Input: dimensioned drawing with shaded views. Units: mm. Origin: part minimum x, y, z. A direction names the side the tool comes from. Round coordinates to 2 decimals unless told otherwise and drop trailing zeros. Loops run counter-clockwise (first coordinate to the right, second up) from the corner with the lowest first, then second, coordinate; pieces in that order, holes last. Notation, with made-up numbers: M 88.5,0.25 L 146.5,0.25 A5 cw 146.5,8.25 Z; hole C 55.25,47 d4. An arc over 180 degrees is marked long. Answer as CSV lines item,"result". Start each with the question number.
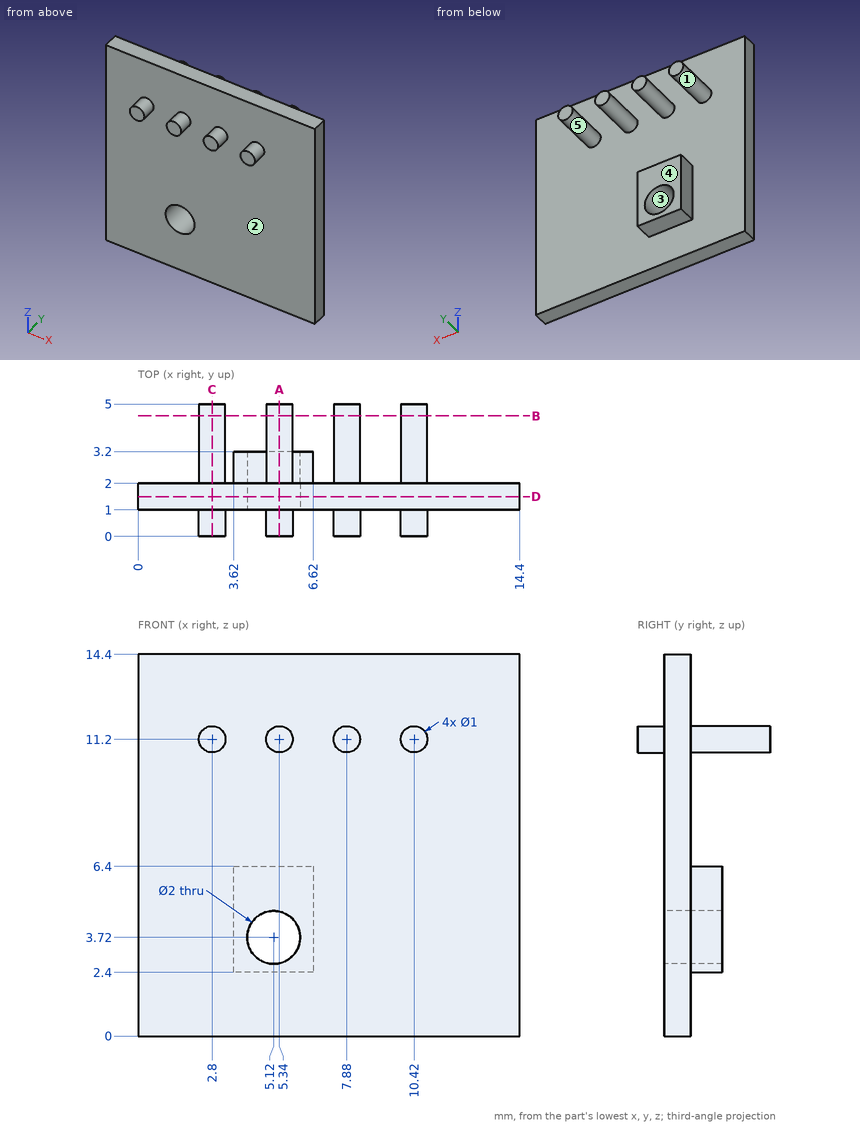
1) Contact query for flat-ended pins moving along their axis: pin 1 Ø1.3 at (y, z) = (3, 4.5) entering from +X; pin 2 Ø3 at (x, y) = (11, 4) entering from +Z; pin 3 Ø1.5 at (x, z) = (11, 3.5) entering from +Y. Output: stop coordinate, or through.
2) Ray query, line 1 along Z through (x, y) = (5.12, 2.1); line 2 along Y through (x, z) = (7, 11); line 3 along Y through (x, z) = (6.5, 5.5). Return the intervals inside material, ascending.
3) Mould query, pull axis Z, two halves, no side actions, for the marked faces 1, 2 and 3. Classes: pulls with the +Z half, pulls with the -Z half, needs draft (parallel to the pull), parting line crosses it, or undercut.
4) Section B-B, the plane y = 4.55. Return loops of the section in (x, z), and give its area (3 significant figures).
5) Access query for the marked faces 4 and 5. Directions: +Z, -Z, +X, -X, +Y, -Y. A direction counts if a zero-diameter tool reaches every point of the face in a straight line with its end or side. Return the directions, or none.
6) Section C-C, the plane x = 2.8. Return loops of the section in (y, z), and give its area (3 significant figures).
7) Section D-D, the plane y = 1.5. Return loops of the section in (x, z), and give its area (3 significant figures).
8) Section A-A, the plane x = 5.34. Return loops of the section in (y, z).
Findings below:
1,pin 1,"x = 6.62"
1,pin 2,"z = 11.7"
1,pin 3,"y = 2"
2,line 1,"2.4 to 2.72, 4.72 to 6.4, 10.75 to 11.65"
2,line 2,"1 to 2"
2,line 3,"1 to 3.2"
3,face 1,"parting line crosses it"
3,face 2,"needs draft"
3,face 3,"undercut"
4,outline,"C 2.8,11.2 d1; C 5.34,11.2 d1; C 7.88,11.2 d1; C 10.42,11.2 d1"
4,area,"3.14 mm²"
5,face 4,"-Z, +X, -X, +Y"
5,face 5,"+Y"
6,outline,"M 0,10.7 L 1,10.7 L 1,0 L 2,0 L 2,10.7 L 5,10.7 L 5,11.7 L 2,11.7 L 2,14.4 L 1,14.4 L 1,11.7 L 0,11.7 Z"
6,area,"18.4 mm²"
7,outline,"M 0,0 L 14.4,0 L 14.4,14.4 L 0,14.4 Z; hole C 5.12,3.72 d2"
7,area,"204 mm²"
8,outline,"M 0,10.7 L 1,10.7 L 1,4.7 L 3.2,4.7 L 3.2,6.4 L 2,6.4 L 2,10.7 L 5,10.7 L 5,11.7 L 2,11.7 L 2,14.4 L 1,14.4 L 1,11.7 L 0,11.7 Z; M 1,0 L 2,0 L 2,2.4 L 3.2,2.4 L 3.2,2.74 L 1,2.74 Z"
